Work out the finished part from the listing and answer in its coordinate system (mm). Face numbers are marked on the shaded views. A direction names the side the tool comes from. Coordinates: 2 decimals unless noted, no trailing zeros. Order: outer loops, then holes, each group sorted by start corner. A loop starts at its lowest first (then second) coordinate and runs counter-clockwise, first axis right, second up.
```python
from build123d import *

# Parameters (mm, degrees)
F0_R     = 95.25
F0_R_2   = 10.31875
F0_R_3   = 12.7
F1_DEPTH = 25.4
F2_DEPTH = 127
F3_R     = 5.08
F4_R     = 7.62


with BuildPart() as f1:
    # F0 (on Front) → F1 (new body)
    with BuildSketch(Plane.XZ):
        Circle(F0_R)
        Circle(F0_R_2, mode=Mode.SUBTRACT)
        with Locations((0, 69.85)):
            Circle(F0_R_3, mode=Mode.SUBTRACT)
    extrude(amount=F1_DEPTH)

    # F0 (on Front) → F2 (join)
    with BuildSketch(Plane.XZ):
        with Locations((0, 69.85)):
            Circle(F0_R_3)
    extrude(amount=F2_DEPTH)

    # F3
    f3_edges = [f1.edges().sort_by_distance(p)[0] for p in [
        (-95.25, -25.4, 0),
        (-95.25, 0, 0),
    ]]
    fillet(f3_edges, radius=F3_R)

    # F4
    f4_edges = [f1.edges().sort_by_distance(p)[0] for p in [
        (-12.7, -127, 69.85),
    ]]
    fillet(f4_edges, radius=F4_R)


solid = f1.part
```
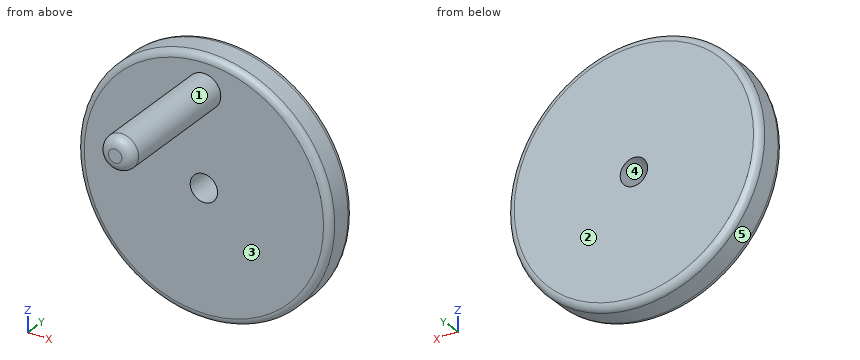
1. Flat-ended cylindrical pins translate along their axes: pin 1 (1.5 mm diameter, centred on x = -7, y = -22, fed in from -Z); pin 2 (10 mm diameter, centred on y = -27, z = -31, fed in from -X); pin 3 (23.5 mm diameter, centred on x = 0, z = 0, fed in from -Y). Find the tip coordinate at first contact, or state that the pin passes through.
2. The part is cut by section A-A (z = 0). Determine the outline of the cut face in (x, y), plus the area to 3 significant figures.
3. The part is cut by section B-B (y = -90). Determine the outline of the cut face in (x, z), plus the area to 3 significant figures.
4. Consider probe 1 along Z at (x, y) = (0, -8); probe 2 along Y at (x, z) = (47, 39); probe 3 along Z at (x, y) = (5, -5.5). Determine where each line is inside the solid, lowest interval first.
5. The mould has two halves that part along Z. Classify the marked faces 3, 4 and 5: released by +Z, released by -Z, zero draft, split by the parting line, or undercut.
6. For the marked faces 1 and 2, determine the directions among +Z, -Z, +X, -X, +Y, -Y from which every point of the face is accessible in a straight line to the end or side of a thin tool.
Worked out:
1. pin 1: stops at z = -94.92
1. pin 2: stops at x = -90.28
1. pin 3: stops at y = -25.4
2. outline: (-95.25, -20.32) arc R5.08 ccw to (-90.17, -25.4) - (-10.32, -25.4) - (-10.32, 0) - (-90.17, 0) arc R5.08 ccw to (-95.25, -5.08) - close; (10.32, -25.4) - (90.17, -25.4) arc R5.08 ccw to (95.25, -20.32) - (95.25, -5.08) arc R5.08 ccw to (90.17, 0) - (10.32, 0) - close
2. area: 4,290 mm2
3. outline: circle Ø25.4 at (0, 69.85)
3. area: 507 mm2
4. probe 1: z = -95.25 to -10.32, 10.32 to 95.25
4. probe 2: y = -25.4 to 0
4. probe 3: z = -95.12 to -9.03, 9.03 to 95.12
5. face 3: zero draft
5. face 4: undercut
5. face 5: split by the parting line
6. face 1: -Y
6. face 2: +Z, -Z, +X, -X, +Y
